from build123d import *

# Parameters (mm, degrees)
SKETCH1_R          = 8
EXTRUDE1_DEPTH     = 366
SKETCH3_R          = 8
SKETCH3_R_2        = 6
CUT_EXTRUDE1_DEPTH = 34
SKETCH4_R          = 8
SKETCH4_R_2        = 6
CUT_EXTRUDE2_DEPTH = 20
SKETCH5_R          = 6
EXTRUDE2_DEPTH     = 10
SKETCH7_R          = 8
SKETCH7_R_2        = 6
EXTRUDE3_DEPTH     = 3
SKETCH8_R          = 8
SKETCH8_R_2        = 6
EXTRUDE4_DEPTH     = 3


with BuildPart() as part:
    # Sketch1 → Extrude1 (new body)
    with BuildSketch(Plane.XY):
        Circle(SKETCH1_R)
    extrude(amount=EXTRUDE1_DEPTH)

    # Sketch3 → Cut-Extrude1 (cut)
    with BuildSketch(Plane.XY.offset(366)):
        Circle(SKETCH3_R)
        Circle(SKETCH3_R_2, mode=Mode.SUBTRACT)
    extrude(amount=-CUT_EXTRUDE1_DEPTH, mode=Mode.SUBTRACT)

    # Sketch4 → Cut-Extrude2 (cut)
    with BuildSketch(Plane(origin=(0, 0, 0), x_dir=(-1, 0, 0), z_dir=(0, 0, -1))):
        Circle(SKETCH4_R)
        Circle(SKETCH4_R_2, mode=Mode.SUBTRACT)
    extrude(amount=-CUT_EXTRUDE2_DEPTH, mode=Mode.SUBTRACT)

    # Sketch5 → Extrude2 (add)
    with BuildSketch(Plane.XY.offset(366)):
        Circle(SKETCH5_R)
    extrude(amount=EXTRUDE2_DEPTH)

    # Sketch7 → Extrude3 (add)
    with BuildSketch(Plane.XY.offset(332)):
        Circle(SKETCH7_R)
        Circle(SKETCH7_R_2, mode=Mode.SUBTRACT)
    extrude(amount=EXTRUDE3_DEPTH)

    # Sketch8 → Extrude4 (add)
    with BuildSketch(Plane(origin=(0, 0, 20), x_dir=(-1, 0, 0), z_dir=(0, 0, -1))):
        Circle(SKETCH8_R)
        Circle(SKETCH8_R_2, mode=Mode.SUBTRACT)
    extrude(amount=EXTRUDE4_DEPTH)


solid = part.part
Check sheet for the modelled part. Datum: model origin and axes. Units: mm. A direction names the side the tool comes from. Round coordinates to 2 decimals unless told otherwise and drop trailing zeros. Loops run counter-clockwise (first coordinate to the right, second up) from the corner with the lowest first, then second, coordinate; pieces in that order, holes last.
1. Set-up check for faces 1 (the cylindrical face through (-6, 0, 356)), 2 (the cylindrical face through (6, 0, 8)), 3 (the flat face through (0, 0, 376)): record each of +Z, -Z, +X, -X, +Y, -Y from which the full face is reachable in a straight line by a thin tool's end or side.
2. Sectioned sample at C-C on z = 26.5. Record the boundary of the cut face in (x, y), and give its area (3 significant figures).
3. Scan lines: probe 1 along X at (y, z) = (-0.5, 174); probe 2 along Z at (x, y) = (-4.25, 5.5); probe 3 along Y at (x, z) = (1, 75). Record each from-to range of solid material in increasing order.
4. Sectioned sample at A-A on x = 0. Record the boundary of the cut face in (y, z).
5. Gauge pin test, flat end, axial feed: pin 1 Ø3 at (x, z) = (6, 187) entering from -Y. Record the tip position at first contact, or that the pin passes through.
Recorded:
1. face 1: +Z
1. face 2: -Z
1. face 3: +Z, +X, -X, +Y, -Y
2. outline: circle Ø16 at (0, 0)
2. area: 201 mm2
3. probe 1: x = -7.98 to 7.98
3. probe 2: z = 17 to 335
3. probe 3: y = -7.94 to 7.94
4. outline: (-8, 17) - (-6, 17) - (-6, 0) - (6, 0) - (6, 17) - (8, 17) - (8, 335) - (6, 335) - (6, 376) - (-6, 376) - (-6, 335) - (-8, 335) - close
5. pin 1: stops at y = -6.61
